```python
from build123d import *

# Parameters (mm, degrees)
PAD_DEPTH    = 80
PAD001_DEPTH = 12.5
PAD002_DEPTH = 12.5
SKETCH003_R  = 32.5
POCKET_DEPTH = 105.001


with BuildPart() as part:
    # Sketch → Pad (new body)
    with BuildSketch(Plane.XZ):
        with BuildLine():
            ThreePointArc((0, -40), (40, 3e-05), (-6.1e-05, 40))
            Line((-52, 40), (-6.1e-05, 40))
            Line((-52, -40), (-52, 40))
            Line((0, -40), (-52, -40))
        make_face()
    extrude(amount=PAD_DEPTH)

    # Sketch001 → Pad001 (new body)
    with BuildSketch(Plane.XZ.offset(80)):
        with BuildLine():
            Line((-60, 48), (-5.9e-05, 48))
            ThreePointArc((-5.9e-05, -48), (48, 0), (-5.9e-05, 48))
            Line((-5.9e-05, -48), (-60, -48))
            Line((-60, -48), (-60, 48))
        make_face()
    extrude(amount=PAD001_DEPTH)

    # Sketch002 → Pad002 (new body)
    with BuildSketch(Plane(origin=(0, 0, 0), x_dir=(1, 0, 0), z_dir=(0, 1, 0))):
        with BuildLine():
            Line((-60, 48), (-5.9e-05, 48))
            ThreePointArc((-5.9e-05, -48), (48, 0), (-5.9e-05, 48))
            Line((-5.9e-05, -48), (-60, -48))
            Line((-60, -48), (-60, 48))
        make_face()
    extrude(amount=PAD002_DEPTH)

    # Sketch003 → Pocket (cut, through all)
    with BuildSketch(Plane(origin=(0, 12.5, 0), x_dir=(1, 0, 0), z_dir=(0, 1, 0))):
        with Locations((-10, 0)):
            Circle(SKETCH003_R)
    extrude(amount=-POCKET_DEPTH, mode=Mode.SUBTRACT)


solid = part.part
```
The model under review builds one solid part; all positions refer to its coordinate system, in mm. A direction names the side the tool comes from. Coordinates: 2 decimals unless noted, no trailing zeros. Write each loop counter-clockwise with the first axis right and the second up, starting at its lowest first coordinate (ties: lowest second). Pieces come first, ordered by that corner, then holes.
1) We need section C-C on y = -52. State the section outline as (x, z) points.
2) We need section B-B on x = -17. State the section outline as (y, z) points, then the cut area to 3 significant figures.
3) Machinability: for faces 5 (the face through (-26, -39, -40)), 6 (the face through (-10, -80, 43)), 7 (the face through (-26, -39, 40)), 8 (the face through (39.99, -39.44, -0.88)), 9 (the face through (-30, -86, -48)), which of the approach directions +Z, -Z, +X, -X, +Y, -Y give a long, thin tool a straight path to every point of the face, cutting with its end or side? Answer none if there is none.
4) We need section D-D on x = -46.5. State the section outline as (y, z) points, then the cut area to 3 significant figures.
5) The part is to be moulded in two halves that separate along Y. For faces 1 (the face through (-10, 0, -43)), 2 (the face through (-52, -39, -1)), 3 (the face through (-5, 12.5, -33)), 4 (the face through (-30, 6, -48)), say which applies: pulls with the +Y half, pulls with the -Y half, needs draft (parallel to the pull), parting line crosses it, or undercut.
6) We need section A-A on z = 0. State the section outline as (x, y) points.
7) Clearance check with flat-ended pins moving along their axes: pin 1 Ø1.5 at (y, z) = (-68.5, 7.5) entering from +X; pin 2 Ø5 at (y, z) = (-64.5, 32) entering from -X; pin 3 Ø3 at (y, z) = (-27, 22.5) entering from +X. State where each tip first meets the part, or that it passes through.
8) To check wall thickness, follow probe 1 along X at (y, z) = (-46.5, 0); probe 2 along Z at (x, y) = (-10, -28); probe 3 along Y at (x, z) = (33, -24). State the ranges of each line that lie inside material, in increasing order.
Answer list:
1. outline: (-52, -40) - (0, -40) arc R40 ccw to (0, 40) - (-52, 40) - close; hole circle Ø65 at (-10, 0)
2. outline: (-92.5, -48) - (-80, -48) - (-80, -40) - (0, -40) - (0, -48) - (12.5, -48) - (12.5, -31.74) - (-92.5, -31.74) - close; (-92.5, 31.74) - (12.5, 31.74) - (12.5, 48) - (0, 48) - (0, 40) - (-80, 40) - (-80, 48) - (-92.5, 48) - close
2. area: 2,140 mm2
3. face 5: -Z, +X, -X
3. face 6: none
3. face 7: +Z, +X, -X
3. face 8: +X
3. face 9: -Z, +X, -X, +Y, -Y
4. outline: (-92.5, -48) - (-80, -48) - (-80, -40) - (0, -40) - (0, -48) - (12.5, -48) - (12.5, 48) - (0, 48) - (0, 40) - (-80, 40) - (-80, 48) - (-92.5, 48) - close
4. area: 8,800 mm2
5. face 1: undercut
5. face 2: undercut
5. face 3: pulls with the +Y half
5. face 4: needs draft
6. outline: (-60, -92.5) - (-42.5, -92.5) - (-42.5, 12.5) - (-60, 12.5) - (-60, 0) - (-52, 0) - (-52, -80) - (-60, -80) - close; (22.5, -92.5) - (48, -92.5) - (48, -80) - (40, -80) - (40, 0) - (48, 0) - (48, 12.5) - (22.5, 12.5) - close
7. pin 1: stops at x = 39.43
7. pin 2: stops at x = -52
7. pin 3: stops at x = 34.04
8. probe 1: x = -52 to -42.5, 22.5 to 40
8. probe 2: z = -40 to -32.5, 32.5 to 40
8. probe 3: y = -92.5 to -80, 0 to 12.5
